from build123d import *

# Parameters (mm, degrees)
SKETCH_1_W          = 50
SKETCH_1_H          = 50
SKETCH_1_R          = 7.5
EXTRUDE_1_DEPTH     = 5
SKETCH_3_R          = 0.75
CUT_EXTRUDE_2_DEPTH = 36.707142143
SKETCH_4_R          = 0.75
CUT_EXTRUDE_3_DEPTH = 36.707142143
SKETCH_5_OUTSIDE_W  = 66.178
SKETCH_5_OUTSIDE_H  = 66.178
SKETCH_5_OUTSIDE_R  = 20
CUT_EXTRUDE_4_DEPTH = 36.707142143


with BuildPart() as part:
    # 草图1 → 凸台-拉伸1 (new body)
    with BuildSketch(Plane(origin=(0, 0, 0), x_dir=(1, 0, 0), z_dir=(0, 1, 0))):
        Rectangle(SKETCH_1_W, SKETCH_1_H)
        with Locations(Location((0, 0, 0), (0, 0, 270))):
            Circle(SKETCH_1_R, mode=Mode.SUBTRACT)
    extrude(amount=EXTRUDE_1_DEPTH)

    # 草图3 → 切除-拉伸2 (cut, through all)
    with BuildSketch(Plane.XZ):
        with Locations(Location((-7, 7, 0), (0, 0, 270))):
            Circle(SKETCH_3_R)
        with Locations(Location((7, 7, 0), (0, 0, 270))):
            Circle(SKETCH_3_R)
        with Locations(Location((7, -7, 0), (0, 0, 270))):
            Circle(SKETCH_3_R)
        with Locations(Location((-7, -7, 0), (0, 0, 270))):
            Circle(SKETCH_3_R)
    extrude(amount=-CUT_EXTRUDE_2_DEPTH, mode=Mode.SUBTRACT)

    # 草图4 → 切除-拉伸3 (cut, through all)
    with BuildSketch(Plane(origin=(0, 5, 0), x_dir=(1, 0, 0), z_dir=(0, 1, 0))):
        with Locations(Location((0, -17.5, 0), (0, 0, 270))):
            Circle(SKETCH_4_R)
        with Locations(Location((0, 17.5, 0), (0, 0, 270))):
            Circle(SKETCH_4_R)
        with Locations(Location((17.5, 0, 0), (0, 0, 270))):
            Circle(SKETCH_4_R)
        with Locations(Location((-17.5, 0, 0), (0, 0, 270))):
            Circle(SKETCH_4_R)
    extrude(amount=-CUT_EXTRUDE_3_DEPTH, mode=Mode.SUBTRACT)

    # 草图5 outside → 切除-拉伸4 (cut, through all)
    with BuildSketch(Plane(origin=(0, 5, 0), x_dir=(1, 0, 0), z_dir=(0, 1, 0))):
        Rectangle(SKETCH_5_OUTSIDE_W, SKETCH_5_OUTSIDE_H)
        with Locations(Location((0, 0, 0), (0, 0, 270))):
            Circle(SKETCH_5_OUTSIDE_R, mode=Mode.SUBTRACT)
    extrude(amount=-CUT_EXTRUDE_4_DEPTH, mode=Mode.SUBTRACT)


solid = part.part
Here's how the part is built. I have some questions about the finished solid (model axes, mm). Round coordinates to 2 decimals unless told otherwise and drop trailing zeros. Loops run counter-clockwise (first coordinate to the right, second up) from the corner with the lowest first, then second, coordinate; pieces in that order, holes last. Notation, with made-up numbers: M 78,15.5 L 102,15.5 A12 cw 102,37.5 Z; hole C 61.5,60.25 d5. An arc over 180 degrees is marked long. Write each question's results on one line, items separated by ' | '. Start each with the question number.
(1) Will these pins go through, and if not, where does the flat tip stop? P1, Ø1, axis at x = 14.5, y = 3, coming from the -Z side; P2, Ø9, axis at x = 0, z = 0, coming from the -Y side; P3, Ø2, axis at x = 12.5, y = 2.5, coming from the -Z side.
(2) I want a section at B-B (y = 3.75). State how many separate pieces and enclosed holes the cut face has, then the cut area to 3 significant figures.
(3) If I drill on probe 1 along X at (y, z) = (1.15, 0); probe 2 along Z at (x, y) = (-5, 2.4); probe 3 along X at (y, z) = (0.75, 3.5), over which ranges is the centre line in solid material (lowest first)? Write a range as from..to.
(4) I want a section at C-C (z = -17.5). Please give me the cut outline in (x, y), then the cut area to 3 significant figures.
(5) Thinking about a two-plate mould opening in X: for faces 1 (the cylindrical face through (-0.456, 2.535, -18.095)), 2 (the flat face through (9, 5, 0)), 3 (the cylindrical face through (-19.524, 2.535, -4.336)), which applies, pulls with the +X half, pulls with the -X half, needs draft (parallel to the pull), parting line crosses it, or undercut?
(6) I want a section at A-A (x = -7). Please give me the cut outline in (y, z) (3 decimals).
(7) I want a section at D-D (z = -7). Please give me the cut outline in (x, y) (3 decimals), then the cut area to 3 significant figures.
Solved:
1) P1: stops at z = -14.28 | P2: passes through | P3: stops at z = -16.36
2) separate pieces: 1 | enclosed holes: 9 | area: 1,070 mm²
3) probe 1: x = -20..-18.25, -16.75..-7.5, 7.5..16.75, 18.25..20 | probe 2: z = -19.36..-5.59, 5.59..19.36 | probe 3: x = -19.69..-6.63, 6.63..19.69
4) outline: M -9.68,0 L -0.75,0 L -0.75,5 L -9.68,5 Z; M 0.75,0 L 9.68,0 L 9.68,5 L 0.75,5 Z | area: 89.3 mm²
5) face 1: undercut | face 2: needs draft | face 3: parting line crosses it
6) outline: M 0,-18.735 L 5,-18.735 L 5,-7.75 L 0,-7.75 Z; M 0,-6.25 L 5,-6.25 L 5,-2.693 L 0,-2.693 Z; M 0,2.693 L 5,2.693 L 5,6.25 L 0,6.25 Z; M 0,7.75 L 5,7.75 L 5,18.735 L 0,18.735 Z
7) outline: M -18.735,0 L -7.75,0 L -7.75,5 L -18.735,5 Z; M -6.25,0 L -2.693,0 L -2.693,5 L -6.25,5 Z; M 2.693,0 L 6.25,0 L 6.25,5 L 2.693,5 Z; M 7.75,0 L 18.735,0 L 18.735,5 L 7.75,5 Z | area: 145 mm²
